Work out the finished part from the listing and answer in its coordinate system (mm). A direction names the side the tool comes from. Round coordinates to 2 decimals unless told otherwise and drop trailing zeros. Order: outer loops, then holes, each group sorted by start corner. A loop starts at its lowest first (then second) coordinate and runs counter-clockwise, first axis right, second up. Notation, with made-up numbers: M 55.5,30.25 L 67.5,30.25 A10 ccw 67.5,38.25 Z; hole C -29,30.5 d7. An arc over 180 degrees is marked long. Return JSON: item names as keys, results as strings.
from build123d import *

# Parameters (mm, degrees)
F0_R     = 45
F1_DEPTH = 19
F2_W     = 7
F2_H     = 5
F2_W_2   = 59
F2_H_2   = 16
F3_DEPTH = 17
F4_W     = 6
F4_H     = 11
F4_W_2   = 11
F4_H_2   = 16
F4_W_3   = 10.7800960541
F4_H_3   = 45.1917052269
F4_R     = 5.5
F5_DEPTH = 19.001
F7_START = -12
F6_W     = 0.7
F6_H     = 5
F7_DEPTH = 5
F8_W     = 20.6779545471
F8_H     = 16
F9_DEPTH = 1.82
F10_SIZE = 2


with BuildPart() as f1:
    # F0 (on Top) → F1 (new body)
    with BuildSketch(Plane.XY):
        Circle(F0_R)
    extrude(amount=F1_DEPTH)

    # F2 (on face) → F3 (cut)
    with BuildSketch(Plane.XY.offset(19)):
        Polygon((41.5, 2.5), (41.5, 8), (3.5, 8), (3.5, -8), (41.5, -8), (41.5, -2.5), align=None)
        with Locations((45, 0)):
            Rectangle(F2_W, F2_H)
        with Locations((0, 18)):
            Rectangle(F2_W_2, F2_H_2)
        with Locations((0, -18)):
            Rectangle(F2_W_2, F2_H_2)
        Polygon((-3.5, 8), (-41.5, 8), (-41.5, 2.5), (-41.5, -2.5), (-41.5, -8), (-3.5, -8), align=None)
        with Locations((-45, 0)):
            Rectangle(F2_W, F2_H)
    extrude(amount=-F3_DEPTH, mode=Mode.SUBTRACT)

    # F4 (on face) → F5 (cut, through all)
    with BuildSketch(Plane.XY.offset(19)):
        with Locations((-34.5, 15.5)):
            Rectangle(F4_W, F4_H)
        with Locations((34.5, 15.5)):
            Rectangle(F4_W, F4_H)
        with Locations((-5.5, 33.5)):
            Rectangle(F4_W, F4_H)
        with Locations((5.5, 33.5)):
            Rectangle(F4_W, F4_H)
        with Locations((-9, 0)):
            Rectangle(F4_W_2, F4_H_2)
        with Locations((9, 0)):
            Rectangle(F4_W_2, F4_H_2)
        with Locations((-47.590048027, 0)):
            Rectangle(F4_W_3, F4_H_3)
        with Locations((47.590048027, 0)):
            Rectangle(F4_W_3, F4_H_3)
        with Locations((0, 18)):
            Circle(F4_R)
        with Locations((0, -18)):
            Circle(F4_R)
    extrude(amount=-F5_DEPTH, mode=Mode.SUBTRACT)

    # F6 (on face) → F7 (join)
    with BuildSketch(Plane.XY.offset(19).offset(F7_START)):
        with Locations((-41.85, 0)):
            Rectangle(F6_W, F6_H)
        with Locations((41.85, 0)):
            Rectangle(F6_W, F6_H)
    extrude(amount=-F7_DEPTH)

    # F8 (on face) → F9 (join)
    with BuildSketch(Plane.XY.offset(2)):
        with Locations((-20.1610227264, 0)):
            Rectangle(F8_W, F8_H)
        with Locations((20.1610227264, 0)):
            Rectangle(F8_W, F8_H)
    extrude(amount=F9_DEPTH)

    # F10
    f10_edges = [f1.edges().sort_by_distance(p)[0] for p in [
        (0, -45, 0),
        (0, 45, 0),
    ]]
    chamfer(f10_edges, length=F10_SIZE)


solid = f1.part
Item 1: Which of the six approach directions +Z, -Z, +X, -X, +Y, -Y give full straight-line access (tool end or side, diameter ignored) to faces 1 (the flat face through (-41.5, -0.1, 6.8)), 2 (the flat face through (3.5, 0, 10)), 3 (the flat face through (-14.5, 0, 1))?
Output:
{"face 1": "+Z", "face 2": "+Z, -Z", "face 3": "-Z"}
Item 2: Find section A-A (x = 0). Determine the outline of the cut face in (y, z).
Output:
{"outline": "M -45,2 L -43,0 L -23.5,0 L -23.5,2 L -26,2 L -26,19 L -45,19 Z; M -12.5,0 L 12.5,0 L 12.5,2 L 10,2 L 10,19 L -10,19 L -10,2 L -12.5,2 Z; M 23.5,0 L 43,0 L 45,2 L 45,19 L 26,19 L 26,2 L 23.5,2 Z"}
Item 3: Consider line 1 along Y through (x, z) = (19.5, 3.75); line 2 along X through (y, z) = (18, 7); line 3 along X through (y, z) = (-15, 8.25). Determine where each line is inside the solid, lowest interval first. Write a range as [from, to].
Output:
{"line 1": "y = [-40.56, -26], [-10, 10], [26, 40.56]", "line 2": "x = [-41.24, -37.5], [-31.5, -29.5], [29.5, 31.5], [37.5, 41.24]", "line 3": "x = [-42.2, -29.5], [29.5, 42.2]"}
Item 4: Each of these flat-tipped pins is pushed along its axis until it touches: pin 1 (1.5 mm diameter, centred on y = -24.5, z = 9.5, fed in from +X); pin 2 (9.5 mm diameter, centred on x = 30, z = 9.5, fed in from +Y); pin 3 (1 mm diameter, centred on x = -28.5, z = 10, fed in from +Y); pin 4 (6.5 mm diameter, centred on x = 0, y = -18, fed in from +Z). Where does it stop, or does it pass through?
Output:
{"pin 1": "stops at x = 38.22", "pin 2": "stops at y = 37.25", "pin 3": "stops at y = 35.23", "pin 4": "passes through"}
Item 5: The mould has two halves that part along Y. Classify faces 4 (the cylindrical face through (-0.766, -44.993, 10.381)), 5 (the cylindrical face through (0.766, 44.993, 10.381)), 6 (the flat face through (0, 10, 11)), 7 (the flat face through (-37.5, 15, 10)): pulls with the +Y half, pulls with the -Y half, needs draft (parallel to the pull), parting line crosses it, or undercut.
Output:
{"face 4": "pulls with the -Y half", "face 5": "pulls with the +Y half", "face 6": "undercut", "face 7": "undercut"}
Item 6: Find section B-B (z = 15.75). State how many separate pieces and enclosed holes the cut face has, plus the area to 3 significant figures.
Output:
{"separate pieces": "1", "enclosed holes": "6", "area": "2,870 mm^2"}
